```python
from build123d import *

# Parameters (mm, degrees)
F0_W     = 80.747418
F0_H     = 9.217742
F1_DEPTH = 127
F2_R     = 5.08
F3_R     = 5.08
F4_R     = 5.08


with BuildPart() as f1:
    # F0 (on Front) → F1 (new body)
    with BuildSketch(Plane.XZ):
        Rectangle(F0_W, F0_H)
    extrude(amount=F1_DEPTH)

    # F2
    f2_edges = [f1.edges().sort_by_distance(p)[0] for p in [
        (0, -127, 4.608871),
    ]]
    fillet(f2_edges, radius=F2_R)

    # F3
    f3_edges = [f1.edges().sort_by_distance(p)[0] for p in [
        (40.373709, -60.96, 4.608871),
    ]]
    fillet(f3_edges, radius=F3_R)

    # F4
    f4_edges = [f1.edges().sort_by_distance(p)[0] for p in [
        (-40.373709, -60.96, 4.608871),
    ]]
    fillet(f4_edges, radius=F4_R)


solid = f1.part
```
CAD build for the part. Positions are in the model's coordinates, mm. Round coordinates to 2 decimals unless told otherwise and drop trailing zeros. Write each loop counter-clockwise with the first axis right and the second up, starting at its lowest first coordinate (ties: lowest second). Pieces come first, ordered by that corner, then holes. Notation, with made-up numbers: (-10.75, 1.5) - (10.25, 1.5) arc R18 cw to (10.25, 25.5) - close; hole circle Ø8 at (-35.75, 83.5). An arc over 180 degrees is marked (long way). Write item = value, one per line. Start each with the question number.
Q1. Drop a flat-ended pin along its axis: pin 1 (4 mm diameter, centred on y = -109.5, z = 0, fed in from -X). Give the stop position or say it passes through.
Q2. Probe L1, parallel to Y at x = -8, z = -0.25; L2, parallel to Y at x = 14, z = 2.5; L3, parallel to X at y = -57, z = 1.5. List the from-to ranges inside material, lowest first. Write a range as from..to.
Q3. Band-saw the part on A-A (z = 3). Give the cut face in (x, y).
Answers below:
q1.pin_1 = -40.37
q2.L1 = -127..0
q2.L2 = -126.04..0
q2.L3 = -39.98..39.98
q3.outline = (-39, -121.92) arc R3.71 ccw to (-35.29, -125.63) - (35.29, -125.63) arc R3.71 ccw to (39, -121.92) - (39, 0) - (-39, 0) - close
